```python
from build123d import *

# Parameters (mm, degrees)
SKETCH1_W                = 30
SKETCH1_H                = 41.5
BOSS_EXTRUDE1_DEPTH      = 40
SKETCH2_W                = 25
SKETCH2_H                = 29
CUT_EXTRUDE1_DEPTH       = 35.5
SKETCH3_W                = 25
SKETCH3_H                = 35.5
CUT_EXTRUDE2_DEPTH       = 19
SKETCH7_W                = 9
SKETCH7_H                = 9
BOSS_EXTRUDE2_DEPTH      = 3.5
SKETCH8_R                = 3
CUT_EXTRUDE3_DEPTH       = 7
BOSS_EXTRUDE3_DEPTH      = 35
SKETCH10_W               = 30
SKETCH10_H               = 31.25
BOSS_EXTRUDE4_DEPTH      = 16
CUT_EXTRUDE4_DEPTH       = 25
SKETCH12_W               = 8
SKETCH12_H               = 17
CUT_EXTRUDE5_DEPTH       = 2.5
SKETCH13_R               = 2.15
CUT_EXTRUDE6_DEPTH       = 10
SKETCH17_W               = 15.75
SKETCH17_H               = 15.75
BOSS_EXTRUDE5_DEPTH      = 22
SKETCH18_R               = 4.445
CUT_EXTRUDE7_DEPTH       = 62.75
SKETCH19_R               = 2.15
CUT_EXTRUDE8_DEPTH       = 5
SKETCH21_R               = 2.15
CUT_EXTRUDE9_DEPTH       = 5
SKETCH23_W               = 8.875
SKETCH23_H               = 91
BOSS_EXTRUDE6_DEPTH      = 5
CUT_EXTRUDE10_REACH      = 122.109
CUT_EXTRUDE10_END_RADIUS = 4.445
SKETCH25_R               = 2.15
CUT_EXTRUDE11_DEPTH      = 119.170427817
SKETCH26_W               = 25
SKETCH26_H               = 2.5
CUT_EXTRUDE12_DEPTH      = 25.25
SKETCH27_W               = 25
SKETCH27_H               = 8
CUT_EXTRUDE13_DEPTH      = 25.25


with BuildPart() as part:
    # Sketch1 → Boss-Extrude1 (new body)
    with BuildSketch(Plane.XY):
        with Locations((15, 20.75)):
            Rectangle(SKETCH1_W, SKETCH1_H)
    extrude(amount=BOSS_EXTRUDE1_DEPTH)

    # Sketch2 → Cut-Extrude1 (cut)
    with BuildSketch(Plane(origin=(0, 41.5, 0), x_dir=(1, 0, 0), z_dir=(0, 1, 0))):
        with Locations((15, -22.75)):
            Rectangle(SKETCH2_W, SKETCH2_H)
    extrude(amount=-CUT_EXTRUDE1_DEPTH, mode=Mode.SUBTRACT)

    # Sketch3 → Cut-Extrude2 (cut)
    with BuildSketch(Plane(origin=(0, 0, 37.25), x_dir=(-1, 0, 0), z_dir=(0, 0, -1))):
        with Locations((-15, 23.75)):
            Rectangle(SKETCH3_W, SKETCH3_H)
    extrude(amount=-CUT_EXTRUDE2_DEPTH, mode=Mode.SUBTRACT)

    # Sketch7 → Boss-Extrude2 (add)
    with BuildSketch(Plane.XZ):
        with Locations((15, -4.5)):
            Rectangle(SKETCH7_W, SKETCH7_H)
    boss_extrude2 = extrude(amount=-BOSS_EXTRUDE2_DEPTH)

    # Sketch8 → Cut-Extrude3 (cut)
    with BuildSketch(Plane(origin=(0, 3.5, 0), x_dir=(1, 0, 0), z_dir=(0, 1, 0))):
        with Locations(Location((15, 4.5, 0), (0, 0, 270))):
            Circle(SKETCH8_R)
    cut_extrude3 = extrude(amount=-CUT_EXTRUDE3_DEPTH, mode=Mode.SUBTRACT)

    # Sketch9 → Boss-Extrude3 (add)
    with BuildSketch(Plane.XY.offset(40)):
        with BuildLine():
            Line((0, 0), (0, 31.25))
            Line((0, 31.25), (4.5, 31.25))
            ThreePointArc((4.5, 31.25), (15, 20.75), (25.5, 31.25))
            Line((25.5, 31.25), (30, 31.25))
            Line((30, 31.25), (30, 0))
            Line((30, 0), (0, 0))
        make_face()
    extrude(amount=BOSS_EXTRUDE3_DEPTH)

    # Sketch10 → Boss-Extrude4 (add)
    with BuildSketch(Plane.XY.offset(75)):
        with Locations((15, 15.625)):
            Rectangle(SKETCH10_W, SKETCH10_H)
    extrude(amount=BOSS_EXTRUDE4_DEPTH)

    # Mirror1: Boss-Extrude2, Cut-Extrude3 across plane
    add(boss_extrude2.mirror(Plane.XY.offset(45.5)))
    add(cut_extrude3.mirror(Plane.XY.offset(45.5)), mode=Mode.SUBTRACT)

    # Sketch11 → Cut-Extrude4 (cut)
    with BuildSketch(Plane.XY.offset(91)):
        with BuildLine():
            Line((11.825, 31.25), (18.175, 31.25))
            ThreePointArc((18.175, 31.25), (15, 28.075), (11.825, 31.25))
        make_face()
    extrude(amount=-CUT_EXTRUDE4_DEPTH, mode=Mode.SUBTRACT)

    # Sketch12 → Cut-Extrude5 (cut)
    with BuildSketch(Plane.ZY.offset(-30)):
        with Locations((14, 33)):
            Rectangle(SKETCH12_W, SKETCH12_H)
    extrude(amount=CUT_EXTRUDE5_DEPTH, mode=Mode.SUBTRACT)

    # Sketch13 → Cut-Extrude6 (cut)
    with BuildSketch(Plane.ZY):
        with Locations((4.265954999, 36.5)):
            Circle(SKETCH13_R)
    cut_extrude6 = extrude(amount=-CUT_EXTRUDE6_DEPTH, mode=Mode.SUBTRACT)

    # Mirror2: Cut-Extrude6 across plane
    add(cut_extrude6.mirror(Plane(origin=(15, 0, 0), x_dir=(0, 0, 1), z_dir=(1, 0, 0))), mode=Mode.SUBTRACT)

    # Sketch17 → Boss-Extrude5 (add)
    with BuildSketch(Plane(origin=(30, 0, 0), x_dir=(0, 0, -1), z_dir=(1, 0, 0))):
        with Locations((-70.625, 18.375)):
            Rectangle(SKETCH17_W, SKETCH17_H)
        with Locations((-34.875, 18.375)):
            Rectangle(SKETCH17_W, SKETCH17_H)
    extrude(amount=BOSS_EXTRUDE5_DEPTH)

    # Sketch18 → Cut-Extrude7 (cut)
    with BuildSketch(Plane.XY.offset(78.5)):
        with Locations(Location((42.5, 18.375, 0), (0, 0, 270))):
            Circle(SKETCH18_R)
    extrude(amount=-CUT_EXTRUDE7_DEPTH, mode=Mode.SUBTRACT)

    # Sketch19 → Cut-Extrude8 (cut)
    with BuildSketch(Plane(origin=(30, 0, 0), x_dir=(0, 0, -1), z_dir=(1, 0, 0))):
        with Locations((-86.486504599, 26.395706225)):
            Circle(SKETCH19_R)
    extrude(amount=-CUT_EXTRUDE8_DEPTH, mode=Mode.SUBTRACT)

    # Sketch21 → Cut-Extrude9 (cut)
    with BuildSketch(Plane.ZY):
        with Locations(Location((86.486504599, 26.395706225, 0), (0, 0, 180))):
            Circle(SKETCH21_R)
    extrude(amount=-CUT_EXTRUDE9_DEPTH, mode=Mode.SUBTRACT)

    # Sketch23 → Boss-Extrude6 (add)
    with BuildSketch(Plane(origin=(0, 0, 0), x_dir=(-1, 0, 0), z_dir=(0, -1, 0))):
        with Locations((-25.5625, -45.5)):
            Rectangle(SKETCH23_W, SKETCH23_H)
        with Locations((-4.4375, -45.5)):
            Rectangle(SKETCH23_W, SKETCH23_H)
    extrude(amount=BOSS_EXTRUDE6_DEPTH)

    # Cut-Extrude10: up to this cylinder (the profile starts outside it)
    cut_extrude10_end = Plane(origin=(42.5, 18.375, 52.75), z_dir=(0, 0, 1)) * Cylinder(CUT_EXTRUDE10_END_RADIUS, 289.858, mode=Mode.PRIVATE)
    # Sketch24 → Cut-Extrude10 (cut, up to the surface)
    with BuildSketch(Plane(origin=(52, 0, 0), x_dir=(0, 0, -1), z_dir=(1, 0, 0)), mode=Mode.PRIVATE) as cut_extrude10_sk1:
        with BuildLine():
            ThreePointArc((-67.975, 18.375), (-70.625, 21.025), (-73.275, 18.375))
            Line((-73.275, 18.375), (-67.975, 18.375))
        make_face()
    cut_extrude10_tool1 = extrude(cut_extrude10_sk1.sketch, amount=-CUT_EXTRUDE10_REACH, mode=Mode.PRIVATE) - cut_extrude10_end
    add(cut_extrude10_tool1.solids().sort_by_distance((52, 19.499695, 70.625))[0], mode=Mode.SUBTRACT)
    # Sketch24 → Cut-Extrude10 (cut, up to the surface)
    with BuildSketch(Plane(origin=(52, 0, 0), x_dir=(0, 0, -1), z_dir=(1, 0, 0)), mode=Mode.PRIVATE) as cut_extrude10_sk2:
        with BuildLine():
            Line((-67.975, 18.375), (-73.275, 18.375))
            ThreePointArc((-73.275, 18.375), (-70.625, 15.725), (-67.975, 18.375))
        make_face()
    cut_extrude10_tool2 = extrude(cut_extrude10_sk2.sketch, amount=-CUT_EXTRUDE10_REACH, mode=Mode.PRIVATE) - cut_extrude10_end
    add(cut_extrude10_tool2.solids().sort_by_distance((52, 17.250305, 70.625))[0], mode=Mode.SUBTRACT)
    # Sketch24 → Cut-Extrude10 (cut, up to the surface)
    with BuildSketch(Plane(origin=(52, 0, 0), x_dir=(0, 0, -1), z_dir=(1, 0, 0)), mode=Mode.PRIVATE) as cut_extrude10_sk3:
        with BuildLine():
            ThreePointArc((-32.225, 18.375), (-34.875, 21.025), (-37.525, 18.375))
            Line((-37.525, 18.375), (-32.225, 18.375))
        make_face()
    cut_extrude10_tool3 = extrude(cut_extrude10_sk3.sketch, amount=-CUT_EXTRUDE10_REACH, mode=Mode.PRIVATE) - cut_extrude10_end
    add(cut_extrude10_tool3.solids().sort_by_distance((52, 19.499695, 34.875))[0], mode=Mode.SUBTRACT)
    # Sketch24 → Cut-Extrude10 (cut, up to the surface)
    with BuildSketch(Plane(origin=(52, 0, 0), x_dir=(0, 0, -1), z_dir=(1, 0, 0)), mode=Mode.PRIVATE) as cut_extrude10_sk4:
        with BuildLine():
            Line((-32.225, 18.375), (-37.525, 18.375))
            ThreePointArc((-37.525, 18.375), (-34.875, 15.725), (-32.225, 18.375))
        make_face()
    cut_extrude10_tool4 = extrude(cut_extrude10_sk4.sketch, amount=-CUT_EXTRUDE10_REACH, mode=Mode.PRIVATE) - cut_extrude10_end
    add(cut_extrude10_tool4.solids().sort_by_distance((52, 17.250305, 34.875))[0], mode=Mode.SUBTRACT)
    # Sketch24 → Cut-Extrude10 (cut, up to the surface)
    with BuildSketch(Plane(origin=(52, 0, 0), x_dir=(0, 0, -1), z_dir=(1, 0, 0)), mode=Mode.PRIVATE) as cut_extrude10_sk5:
        with BuildLine():
            ThreePointArc((-32.225, 18.375), (-34.875, 21.025), (-37.525, 18.375))
            Line((-37.525, 18.375), (-32.225, 18.375))
        make_face()
    cut_extrude10_tool5 = extrude(cut_extrude10_sk5.sketch, amount=-CUT_EXTRUDE10_REACH, mode=Mode.PRIVATE) - cut_extrude10_end
    add(cut_extrude10_tool5.solids().sort_by_distance((52, 19.499695, 34.875))[0], mode=Mode.SUBTRACT)
    # Sketch24 → Cut-Extrude10 (cut, up to the surface)
    with BuildSketch(Plane(origin=(52, 0, 0), x_dir=(0, 0, -1), z_dir=(1, 0, 0)), mode=Mode.PRIVATE) as cut_extrude10_sk6:
        with BuildLine():
            Line((-32.225, 18.375), (-37.525, 18.375))
            ThreePointArc((-37.525, 18.375), (-34.875, 15.725), (-32.225, 18.375))
        make_face()
    cut_extrude10_tool6 = extrude(cut_extrude10_sk6.sketch, amount=-CUT_EXTRUDE10_REACH, mode=Mode.PRIVATE) - cut_extrude10_end
    add(cut_extrude10_tool6.solids().sort_by_distance((52, 17.250305, 34.875))[0], mode=Mode.SUBTRACT)
    # Sketch24 → Cut-Extrude10 (cut, up to the surface)
    with BuildSketch(Plane(origin=(52, 0, 0), x_dir=(0, 0, -1), z_dir=(1, 0, 0)), mode=Mode.PRIVATE) as cut_extrude10_sk7:
        with BuildLine():
            ThreePointArc((-67.975, 18.375), (-70.625, 21.025), (-73.275, 18.375))
            Line((-73.275, 18.375), (-67.975, 18.375))
        make_face()
    cut_extrude10_tool7 = extrude(cut_extrude10_sk7.sketch, amount=-CUT_EXTRUDE10_REACH, mode=Mode.PRIVATE) - cut_extrude10_end
    add(cut_extrude10_tool7.solids().sort_by_distance((52, 19.499695, 70.625))[0], mode=Mode.SUBTRACT)
    # Sketch24 → Cut-Extrude10 (cut, up to the surface)
    with BuildSketch(Plane(origin=(52, 0, 0), x_dir=(0, 0, -1), z_dir=(1, 0, 0)), mode=Mode.PRIVATE) as cut_extrude10_sk8:
        with BuildLine():
            Line((-67.975, 18.375), (-73.275, 18.375))
            ThreePointArc((-73.275, 18.375), (-70.625, 15.725), (-67.975, 18.375))
        make_face()
    cut_extrude10_tool8 = extrude(cut_extrude10_sk8.sketch, amount=-CUT_EXTRUDE10_REACH, mode=Mode.PRIVATE) - cut_extrude10_end
    add(cut_extrude10_tool8.solids().sort_by_distance((52, 17.250305, 70.625))[0], mode=Mode.SUBTRACT)

    # Sketch25 → Cut-Extrude11 (cut, through all)
    with BuildSketch(Plane(origin=(0, 6, 0), x_dir=(1, 0, 0), z_dir=(0, 1, 0))):
        with Locations(Location((15, -16, 0), (0, 0, 270))):
            Circle(SKETCH25_R)
        with Locations(Location((15, -31, 0), (0, 0, 270))):
            Circle(SKETCH25_R)
    extrude(amount=-CUT_EXTRUDE11_DEPTH, mode=Mode.SUBTRACT)

    # Sketch26 → Cut-Extrude12 (cut)
    with BuildSketch(Plane(origin=(0, 31.25, 0), x_dir=(1, 0, 0), z_dir=(0, 1, 0))):
        with Locations((15, -41.25)):
            Rectangle(SKETCH26_W, SKETCH26_H)
    extrude(amount=-CUT_EXTRUDE12_DEPTH, mode=Mode.SUBTRACT)

    # Sketch27 → Cut-Extrude13 (cut)
    with BuildSketch(Plane(origin=(0, 31.25, 0), x_dir=(1, 0, 0), z_dir=(0, 1, 0))):
        with Locations((15, -46.5)):
            Rectangle(SKETCH27_W, SKETCH27_H)
    extrude(amount=-CUT_EXTRUDE13_DEPTH, mode=Mode.SUBTRACT)


solid = part.part
```
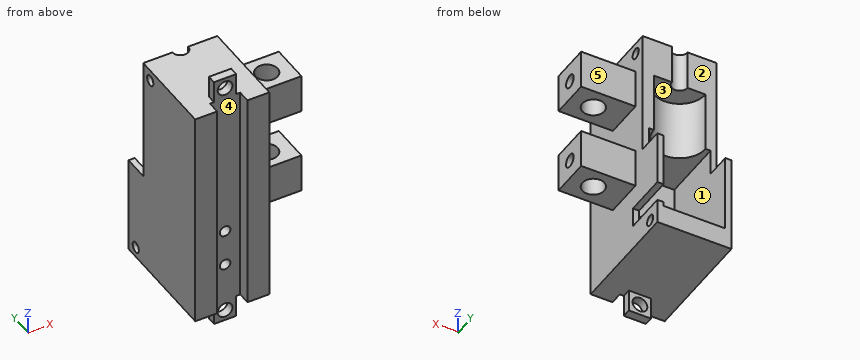
Design review of the part built by this model. Coordinates are the model's own, in mm. Face numbers are marked on the shaded views. A direction names the side the tool comes from. Give positions to 0.01 mm unless a question says otherwise; leave off trailing zeros. Write each loop counter-clockwise with the first axis right and the second up, starting at its lowest first coordinate (ties: lowest second). Pieces come first, ordered by that corner, then holes. Notation, with made-up numbers: (-29.75, 30.5) - (-19.75, 30.5) arc R31 cw to (-19.75, 68.5) - close; hole circle Ø1 at (55, 69). An arc over 180 degrees is marked (long way). Return JSON: item names as keys, results as strings. Group by question number.
(1) We need section D-D, the plane y = 12. Give the boundary of the cut face in (x, z).
(2) We need section A-A, the plane x = 15. Give the number of separate pieces and of enclosed holes in the cut face, then the cut area to 3 significant figures.
(3) Insertion check: pin 1 (11.5 mm diameter, centred on x = 42.5, y = 18.375, fed in from -Z); pin 2 (2 mm diameter, centred on x = 11, z = 39, fed in from -Y); pin 3 (10 mm diameter, centred on x = 32.5, y = 15.5, fed in from -Z); pin 4 (2 mm diameter, centred on y = 36, z = 41.5, fed in from +X). Each pin has a flat end and moves straight along its axis. Give the tip position at first contact, or say it passes through.
(4) We need section B-B, the plane z = 95.5. Give the boundary of the cut face in (x, y).
(5) Mouldability with a two-part tool opening along Z and no side actions: class the marked faces 1 and 2 as +Z half, -Z half, draft (parallel to the pull), parting line (faces both ways), or undercut.
(6) To check wall thickness, follow probe 1 along Z at (x, y) = (23, 22); probe 2 along Z at (x, y) = (5, 30.5); probe 3 along X at (y, z) = (3.7, 31). State the ranges of each line that lie inside material, in increasing order.
(7) Machinability: for the marked faces 3, 4 and 5, which of the approach directions +Z, -Z, +X, -X, +Y, -Y give a long, thin tool a straight path to every point of the face, cutting with its end or side? Answer none if there is none.
(8) We need section C-C, the plane x = 42.5. Give the boundary of the cut face in (y, z), then the cut area to 3 significant figures.
Reported:
{
 "1": {"outline": "(0, 0) - (30, 0) - (30, 27) - (52, 27) - (52, 42.75) - (30, 42.75) - (30, 62.75) - (52, 62.75) - (52, 78.5) - (30, 78.5) - (30, 91) - (0, 91) - close; hole (2.5, 8.25) - (27.5, 8.25) - (27.5, 50.5) - (2.5, 50.5) - close"},
 "2": {"separate pieces": "5", "enclosed holes": "0", "area": "1,520 mm2"},
 "3": {"pin 1": "stops at z = 27", "pin 2": "stops at y = 0", "pin 3": "stops at z = 0", "pin 4": "passes through"},
 "4": {"outline": "(10.5, 0) - (12, 0) - (12, 3.5) - (10.5, 3.5) - close; (18, 0) - (19.5, 0) - (19.5, 3.5) - (18, 3.5) - close"},
 "5": {"face 1": "undercut", "face 2": "draft"},
 "6": {"probe 1": "z = 0 to 8.25, 50.5 to 91", "probe 2": "z = 0 to 8.25, 75 to 91", "probe 3": "x = 0 to 12.85, 17.15 to 30"},
 "7": {"face 3": "+Y", "face 4": "+Z, -Z, -Y", "face 5": "+Z, -Z, +X, +Y"},
 "8": {"outline": "(10.5, 27) - (13.93, 27) - (13.93, 42.75) - (10.5, 42.75) - close; (10.5, 62.75) - (13.93, 62.75) - (13.93, 78.5) - (10.5, 78.5) - close; (22.82, 27) - (26.25, 27) - (26.25, 42.75) - (22.82, 42.75) - close; (22.82, 62.75) - (26.25, 62.75) - (26.25, 78.5) - (22.82, 78.5) - close", "area": "216 mm2"}
}
